from build123d import *

# Parameters (mm, degrees)
SKETCH_1_R      = 2.1
SKETCH_1_R_2    = 8
EXTRUDE_1_DEPTH = 3


with BuildPart() as part:
    # 草图1 → 拉伸1 (new body)
    with BuildSketch(Plane.XY):
        with BuildLine():
            Line((-150, 0), (-125.000376699, 0))
            Line((-125.000376699, 0), (-125.000376699, 39.69983712))
            Line((-125.000376699, 39.69983712), (-113.000376699, 39.69983712))
            Line((-113.000376699, 39.69983712), (-113.000376699, 97.69983712))
            Line((-113.000376699, 97.69983712), (-125.000376699, 97.69983712))
            Line((-125.000376699, 97.69983712), (-125.000376699, 136.962885218))
            Line((-125.000376699, 136.962885218), (-149.291861287, 136.962885218))
            Line((-149.291861287, 136.962885218), (-149.291861287, 159.962885218))
            Line((-149.291861287, 159.962885218), (-55, 190.24809041))
            Line((-55, 190.24809041), (54.687657428, 190.24809041))
            Line((54.687657428, 190.24809041), (149.291861287, 159.962885218))
            Line((149.291861287, 159.962885218), (149.291861287, 136.962885218))
            Line((149.291861287, 136.962885218), (125.000376699, 136.962885218))
            Line((125.000376699, 136.962885218), (125.000376699, 97.69983712))
            Line((125.000376699, 97.69983712), (113.000376699, 97.69983712))
            Line((113.000376699, 97.69983712), (113.000376699, 39.69983712))
            Line((113.000376699, 39.69983712), (125.000376699, 39.69983712))
            Line((125.000376699, 39.69983712), (125.000376699, 0))
            Line((125.000376699, 0), (150, 0))
            ThreePointArc((150, 0), (0, -150), (-150, 0))
        make_face()
        with Locations((-92.750376699, 77.7)):
            Circle(SKETCH_1_R, mode=Mode.SUBTRACT)
        with Locations(Location((-92.750376699, 59.7, 0), (0, 0, 180))):
            Circle(SKETCH_1_R, mode=Mode.SUBTRACT)
        with Locations((-53.5, -83)):
            Circle(SKETCH_1_R, mode=Mode.SUBTRACT)
        with Locations(Location((-53.5, -107, 0), (0, 0, 180))):
            Circle(SKETCH_1_R, mode=Mode.SUBTRACT)
        with Locations((53.5, -107)):
            Circle(SKETCH_1_R, mode=Mode.SUBTRACT)
        with Locations(Location((53.5, -83, 0), (0, 0, 180))):
            Circle(SKETCH_1_R, mode=Mode.SUBTRACT)
        with Locations((-79.250376699, 59.7)):
            Circle(SKETCH_1_R, mode=Mode.SUBTRACT)
        with Locations(Location((-79.250376699, 77.7, 0), (0, 0, 180))):
            Circle(SKETCH_1_R, mode=Mode.SUBTRACT)
        with Locations(Location((79.250376699, 59.7, 0), (0, 0, 180))):
            Circle(SKETCH_1_R, mode=Mode.SUBTRACT)
        with Locations((92.750376699, 59.7)):
            Circle(SKETCH_1_R, mode=Mode.SUBTRACT)
        with Locations((79.250376699, 77.7)):
            Circle(SKETCH_1_R, mode=Mode.SUBTRACT)
        with Locations(Location((92.750376699, 77.7, 0), (0, 0, 180))):
            Circle(SKETCH_1_R, mode=Mode.SUBTRACT)
        Circle(SKETCH_1_R_2, mode=Mode.SUBTRACT)
        with Locations((-58.324201506, -124.520480318)):
            Circle(SKETCH_1_R, mode=Mode.SUBTRACT)
        with Locations(Location((-78.675798494, -112.770480318, 0), (0, 0, 180))):
            Circle(SKETCH_1_R, mode=Mode.SUBTRACT)
        with Locations((-112.770480318, -78.675798494)):
            Circle(SKETCH_1_R, mode=Mode.SUBTRACT)
        with Locations(Location((-124.520480318, -58.324201506, 0), (0, 0, 180))):
            Circle(SKETCH_1_R, mode=Mode.SUBTRACT)
        with Locations((-78.675798494, 112.770480318)):
            Circle(SKETCH_1_R, mode=Mode.SUBTRACT)
        with Locations(Location((-58.324201506, 124.520480318, 0), (0, 0, 180))):
            Circle(SKETCH_1_R, mode=Mode.SUBTRACT)
        with Locations((-11.75, 137)):
            Circle(SKETCH_1_R, mode=Mode.SUBTRACT)
        with Locations(Location((11.75, 137, 0), (0, 0, 180))):
            Circle(SKETCH_1_R, mode=Mode.SUBTRACT)
        with Locations((58.324201506, 124.520480318)):
            Circle(SKETCH_1_R, mode=Mode.SUBTRACT)
        with Locations(Location((78.675798494, 112.770480318, 0), (0, 0, 180))):
            Circle(SKETCH_1_R, mode=Mode.SUBTRACT)
        with Locations((124.520480318, -58.324201506)):
            Circle(SKETCH_1_R, mode=Mode.SUBTRACT)
        with Locations(Location((112.770480318, -78.675798494, 0), (0, 0, 180))):
            Circle(SKETCH_1_R, mode=Mode.SUBTRACT)
        with Locations((78.675798494, -112.770480318)):
            Circle(SKETCH_1_R, mode=Mode.SUBTRACT)
        with Locations(Location((58.324201506, -124.520480318, 0), (0, 0, 180))):
            Circle(SKETCH_1_R, mode=Mode.SUBTRACT)
        with BuildLine():
            Line((42.5, -95), (42.5, -65))
            ThreePointArc((42.5, -65), (39.571067812, -57.928932188), (32.5, -55))
            Line((32.5, -55), (-32.5, -55))
            ThreePointArc((-32.5, -55), (-39.571067812, -57.928932188), (-42.5, -65))
            Line((-42.5, -65), (-42.5, -95))
            Line((-42.5, -95), (-42.5, -125))
            ThreePointArc((-42.5, -125), (-39.571067812, -132.071067812), (-32.5, -135))
            Line((-32.5, -135), (32.5, -135))
            ThreePointArc((32.5, -135), (39.571067812, -132.071067812), (42.5, -125))
            Line((42.5, -125), (42.5, -95))
        make_face(mode=Mode.SUBTRACT)
    extrude(amount=EXTRUDE_1_DEPTH)


solid = part.part
Source: CAD feature listing. Evaluate the final solid. Frame: model axes, mm. A direction names the side the tool comes from. Give positions to 0.01 mm unless a question says otherwise; leave off trailing zeros. Order: outer loops, then holes, each group sorted by start corner. A loop starts at its lowest first (then second) coordinate and runs counter-clockwise, first axis right, second up. Notation, with made-up numbers: (64, 5) -> (76, 5) arc R28 ccw to (76, 40) -> close; hole circle Ø5 at (37.5, 74.5). An arc over 180 degrees is marked (long way). Write item = value, one per line.
Q1. Cut plane B-B, the plane z = 0.5. State how many separate pieces and enclosed holes the cut face has, and give its area (3 significant figures).
Data:
separate_pieces = 1
enclosed_holes = 28
area = 74,000 mm^2
Q2. Material intervals for line 1 (Y direction, x = 5, z = 2.7) (3 decimals); line 2 (Y direction, x = -93.5, z = 0.5); line 3 (X direction, y = -111.5, z = 1.35), sorted ascending. Write a range as from..to.
Data:
line_1 = -149.917..-135, -55..-6.245, 6.245..190.248
line_2 = -117.29..57.74, 61.66..75.74, 79.66..177.88
line_3 = -100.34..-80.35, -77..-42.5, 42.5..77, 80.35..100.34
Q3. Cut plane C-C, the plane x = 104. Output: boundary loops of the cut face in (y, z), and give its area (3 significant figures).
Data:
outline = (-108.09, 0) -> (174.46, 0) -> (174.46, 3) -> (-108.09, 3) -> close
area = 848 mm^2
Q4. Cut plane A-A, the plane y = 44. Output: boundary loops of the cut face in (x, z), and give its area (3 significant figures).
Data:
outline = (-113, 0) -> (113, 0) -> (113, 3) -> (-113, 3) -> close
area = 678 mm^2
Q5. Pull-direction query (X, two-part tool) for faces 1 (the face through (2, 23, 0)), 2 (the face through (3.298, -149.964, 1.479)), 3 (the face through (39.49, -132.15, 1.48)), 4 (the face through (-102.806, 174.893, 1.479)); classes: released by +X, released by -X, zero draft, split by the parting line, or undercut.
Data:
face_1 = zero draft
face_2 = split by the parting line
face_3 = undercut
face_4 = released by -X
Q6. Pin query (flat end, axial travel): pin 1 (6.5 mm diameter, centred on x = -53.5, y = -83, fed in from -Z); pin 2 (1.5 mm diameter, centred on y = -91, z = 1.5, fed in from +X). Return the tip coordinate at first contact, or that it passes through.
Data:
pin_1 = 0
pin_2 = 119.81
Q7. Set-up query: faces 5 (the face through (39.65, -58.01, 1.48)), 6 (the face through (101.328, 175.317, 1.479)). Return all of +Z, -Z, +X, -X, +Y, -Y with unobstructed straight access to the full face (end or side cutting, diameter ignored); none if empty.
Data:
face_5 = +Z, -Z
face_6 = +Z, -Z, +X, +Y
